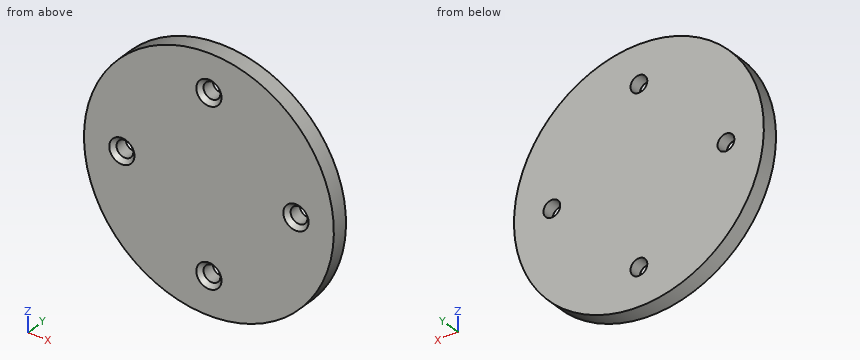
from build123d import *

# Parameters (mm, degrees)
SKETCH1_R                 = 14.875
BOSS_EXTRUDE1_DEPTH       = 2
F_2_0MM_DOWEL_HOLE1_D     = 2
F_2_0MM_DOWEL_HOLE1_DEPTH = 42.93
F_2_0MM_DOWEL_HOLE1_TIP   = 0.600860619
CHAMFER1_SIZE             = 0.5


with BuildPart() as part:
    # Sketch1 → Boss-Extrude1 (new body)
    with BuildSketch(Plane(origin=(0, 0, 0), x_dir=(1, 0, 0), z_dir=(0, 1, 0))):
        with Locations(Location((0, 0, 0), (0, 0, 270))):
            Circle(SKETCH1_R)
    extrude(amount=BOSS_EXTRUDE1_DEPTH)

    # Ø2.0mm Dowel Hole1
    with Locations(Plane(origin=(0, 2, 0), x_dir=(1, 0, 0), z_dir=(0, 1, 0))):
        with Locations((0, 10.365), (10.365, 0), (0, -10.365), (-10.365, 0)):
            Hole(F_2_0MM_DOWEL_HOLE1_D / 2, depth=F_2_0MM_DOWEL_HOLE1_DEPTH)
            with Locations((0, 0, -(F_2_0MM_DOWEL_HOLE1_DEPTH + F_2_0MM_DOWEL_HOLE1_TIP / 2))):  # 118° drill point
                Cone(0, F_2_0MM_DOWEL_HOLE1_D / 2, F_2_0MM_DOWEL_HOLE1_TIP, mode=Mode.SUBTRACT)

    # Chamfer1
    chamfer1_edges = [part.edges().sort_by_distance(p)[0] for p in [
        (1, 0, 10.365),
        (11.365, 0, 0),
        (1, 0, -10.365),
        (-9.365, 0, 0),
    ]]
    chamfer(chamfer1_edges, length=CHAMFER1_SIZE)


solid = part.part
For this review, take the finished solid that the model builds, in its own axes (mm). Round coordinates to 2 decimals unless told otherwise and drop trailing zeros. Order: outer loops, then holes, each group sorted by start corner. A loop starts at its lowest first (then second) coordinate and runs counter-clockwise, first axis right, second up. Notation, with made-up numbers: (40.5, -37) -> (65.5, -37) arc R21 cw to (65.5, 1) -> close; hole circle Ø11 at (87, 36.5). An arc over 180 degrees is marked (long way). Write item = value, one per line. Start each with the question number.
1) Take a section at C-C on y = 1.6. State the section outline as (x, z) points (3 decimals).
2) Take a section at B-B on z = 0. State the section outline as (x, y) points (3 decimals).
3) Insertion check: pin 1 (1.6 mm diameter, centred on x = 0, z = 10.365, fed in from +Y); pin 2 (2.5 mm diameter, centred on x = -10.365, z = 0, fed in from -Y). Each pin has a flat end and moves straight along its axis. Give the tip position at first contact, or say it passes through.
4) Take a section at A-A on x = 0. State the section outline as (y, z) points (3 decimals).
5) Take a section at D-D on x = 8.5. State the section outline as (y, z) points.
6) To check wall thickness, follow line 1 (X direction, y = 0.95, z = 0) (3 decimals); line 2 (Z direction, x = 10.25, y = 0.6); line 3 (Y direction, x = 1, z = 9.25). State the ranges of each line that lie inside material, in increasing order. Write a range as from..to.
Verdict:
q1.outline = circle Ø29.75 at (0, 0); hole circle Ø2 at (-10.365, 0); hole circle Ø2 at (0, -10.365); hole circle Ø2 at (0, 10.365); hole circle Ø2 at (10.365, 0)
q2.outline = (-14.875, 0) -> (-11.865, 0) -> (-11.365, 0.5) -> (-11.365, 2) -> (-14.875, 2) -> close; (-9.365, 0.5) -> (-8.865, 0) -> (8.865, 0) -> (9.365, 0.5) -> (9.365, 2) -> (-9.365, 2) -> close; (11.365, 0.5) -> (11.865, 0) -> (14.875, 0) -> (14.875, 2) -> (11.365, 2) -> close
q3.pin_1 = through
q3.pin_2 = 0.25
q4.outline = (0, -14.875) -> (2, -14.875) -> (2, -11.365) -> (0.5, -11.365) -> (0, -11.865) -> close; (0, -8.865) -> (0.5, -9.365) -> (2, -9.365) -> (2, 9.365) -> (0.5, 9.365) -> (0, 8.865) -> close; (0, 11.865) -> (0.5, 11.365) -> (2, 11.365) -> (2, 14.875) -> (0, 14.875) -> close
q5.outline = (0, -12.21) -> (2, -12.21) -> (2, 12.21) -> (0, 12.21) -> close
q6.line_1 = -14.875..-11.365, -9.365..9.365, 11.365..14.875
q6.line_2 = -10.78..-0.99, 0.99..10.78
q6.line_3 = 0..2
